Verification items for the finished model (mm, model axes). Face numbers are marked on the shaded views. Coordinates: 2 decimals unless noted, no trailing zeros. Order: outer loops, then holes, each group sorted by start corner. A loop starts at its lowest first (then second) coordinate and runs counter-clockwise, first axis right, second up. Notation, with made-up numbers: M 40.5,2 L 64.5,2 A29 cw 64.5,23 Z; hole C -11,60.25 d3. An arc over 180 degrees is marked long. Return JSON: item names as keys, results as strings. Group by question number.
Q1. Mould release check, pull along Z, two halves, no side actions. Record for the marked faces 1, 2 and 3: pulls with the +Z half, pulls with the -Z half, needs draft (parallel to the pull), parting line crosses it, or undercut.
Q2. Section check B-B, the plane z = 8.25. Enter the section's corners in (x, y).
Q3. Go/stop test with flat-tipped pins: pin 1 Ø20 at (x, y) = (0, 0) entering from +Z; pin 2 Ø5 at (y, z) = (-9, 3.5) entering from -X; pin 3 Ø8 at (x, y) = (5.5, -9) entering from +Z; pin 4 Ø2 at (x, z) = (13, 2) entering from +Y. Record where each tip stops, or that it passes through.
Q4. Thickness scan on probe 1 along Z at (x, y) = (13, 0); probe 2 along Y at (x, z) = (0, 8.5); probe 3 along Y at (x, z) = (2.5, 2.5). Record the ranges inside material, lowest first.
Q5. Section check D-D, the plane z = 11. Enter the section's corners in (x, y), then the cut area to 3 significant figures.
Q6. Section check C-C, the plane x = 12.5. Enter the section's corners in (y, z), then the cut area to 3 significant figures.
Q7. Section check A-A, the plane x = 0. Enter the section's corners in (y, z), then the cut area to 3 significant figures.
from build123d import *

# Parameters (mm, degrees)
F0_R      = 17.0053
F1_DEPTH  = 12.319
F3_DEPTH  = 25.4
F3_FACE_R = 3.5052
F4_DEPTH  = 25.4
F5_R      = 11.107827
F6_DEPTH  = 25.4


with BuildPart() as f1:
    # F0 (on Top) → F1 (new body)
    with BuildSketch(Plane.XY):
        Circle(F0_R)
    extrude(amount=F1_DEPTH)

    # F2 (on Right) → F3 (cut)
    with BuildSketch(Plane.YZ):
        with BuildLine():
            ThreePointArc((0, 9.508782), (-3.5052, 6.003582), (0, 2.498382))
            Line((0, 2.498382), (0, 6.003582))
            Line((0, 6.003582), (0, 9.508782))
        make_face()
        with BuildLine():
            Line((0, 6.003582), (0, 2.498382))
            ThreePointArc((0, 2.498382), (2.478551, 3.525031), (3.5052, 6.003582))
            ThreePointArc((3.5052, 6.003582), (2.478551, 8.482132), (0, 9.508782))
            Line((0, 9.508782), (0, 6.003582))
        make_face()
    extrude(amount=-F3_DEPTH, mode=Mode.SUBTRACT)

    # F3_face (on face) → F4 (cut)
    with BuildSketch(Plane(origin=(0, 0, 6.003582), x_dir=(0, 1, 0), z_dir=(-1, 0, 0))):
        Circle(F3_FACE_R)
    extrude(amount=-F4_DEPTH, mode=Mode.SUBTRACT)

    # F5 (on face) → F6 (cut)
    with BuildSketch(Plane(origin=(0, 0, 0), x_dir=(1, 0, 0), z_dir=(0, 0, -1))):
        Circle(F5_R)
    extrude(amount=-F6_DEPTH, mode=Mode.SUBTRACT)


solid = f1.part
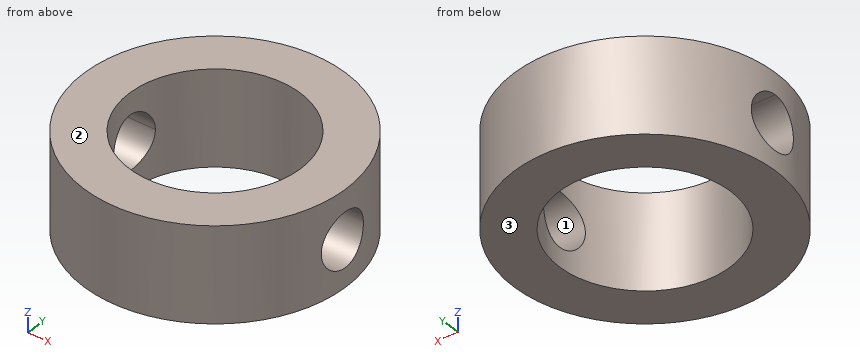
Numbers:
{
 "1": {"face 1": "undercut", "face 2": "pulls with the +Z half", "face 3": "pulls with the -Z half"},
 "2": {"outline": "M -16.79,-2.69 A17.01 ccw 16.79,-2.69 L 10.78,-2.69 A11.11 cw -10.78,-2.69 Z; M -16.79,2.69 L -10.78,2.69 A11.11 cw 10.78,2.69 L 16.79,2.69 A17.01 ccw Z"},
 "3": {"pin 1": "passes through", "pin 2": "stops at x = -15.71", "pin 3": "stops at z = 12.32", "pin 4": "stops at y = 12.05"},
 "4": {"probe 1": "z = 0 to 2.5, 9.51 to 12.32", "probe 2": "y = -17.01 to -11.11, 11.11 to 17.01", "probe 3": "y = -16.82 to -10.82, 10.82 to 16.82"},
 "5": {"outline": "C 0,0 d34.01; hole C 0,0 d22.22", "area": "521 mm2"},
 "6": {"outline": "M -11.53,0 L 11.53,0 L 11.53,12.32 L -11.53,12.32 Z; hole C 0,6 d7.01", "area": "245 mm2"},
 "7": {"outline": "M -17.01,0 L -11.11,0 L -11.11,12.32 L -17.01,12.32 Z; M 11.11,0 L 17.01,0 L 17.01,12.32 L 11.11,12.32 Z", "area": "145 mm2"}
}
